from build123d import *

# Parameters (mm, degrees)
F1_DEPTH = 25.4
F3_DEPTH = 12.7
F5_DEPTH = 12.7


with BuildPart() as f1:
    # F0 (on Front) → F1 (new body)
    with BuildSketch(Plane.XZ):
        Polygon((69.85, 127), (19.05, 127), (0, 127), (0, 0), (39.624, 0), (44.45, 0), (79.248, 0), (79.248, 127), align=None)
    extrude(amount=F1_DEPTH)

    # F2 (on face) → F3 (join)
    with BuildSketch(Plane.XZ.offset(25.4)):
        with BuildLine():
            ThreePointArc((39.624, 97.79), (44.114128, 99.649872), (45.974, 104.14))
            ThreePointArc((45.974, 104.14), (35.133872, 108.630128), (39.624, 97.79))
        make_face()
    extrude(amount=F3_DEPTH)

    # F4 (on face) → F5 (cut)
    with BuildSketch(Plane(origin=(0, 0, 0), x_dir=(1, 0, 0), z_dir=(0, 0, -1))):
        with BuildLine():
            Line((16.637, 12.7), (19.812, 12.7))
            Line((19.812, 12.7), (22.987, 12.7))
            ThreePointArc((22.987, 12.7), (19.812, 15.875), (16.637, 12.7))
        make_face()
        with BuildLine():
            Line((22.987, 12.7), (19.812, 12.7))
            Line((19.812, 12.7), (16.637, 12.7))
            ThreePointArc((16.637, 12.7), (19.812, 9.525), (22.987, 12.7))
        make_face()
        with BuildLine():
            ThreePointArc((62.611, 12.7), (59.436, 15.875), (56.261, 12.7))
            Line((56.261, 12.7), (59.436, 12.7))
            Line((59.436, 12.7), (62.611, 12.7))
        make_face()
        with BuildLine():
            Line((59.436, 12.7), (56.261, 12.7))
            ThreePointArc((56.261, 12.7), (59.436, 9.525), (62.611, 12.7))
            Line((62.611, 12.7), (59.436, 12.7))
        make_face()
    extrude(amount=-F5_DEPTH, mode=Mode.SUBTRACT)


solid = f1.part
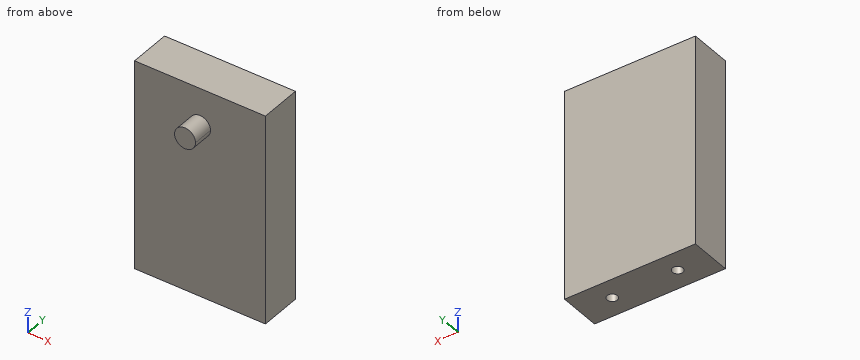
Could you check a few things on this model? Use its own coordinates, in mm. Coordinates: 2 decimals unless noted, no trailing zeros. Loops run counter-clockwise (first coordinate to the right, second up) from the corner with the lowest first, then second, coordinate; pieces in that order, holes last. Notation, with made-up numbers: (35.5, 10.25) -> (43.5, 10.25) arc R25 ccw to (43.5, 34.25) -> close; hole circle Ø6 at (72, 34). An arc over 180 degrees is marked (long way). Answer in a Markdown table with one row per item.
(1) Imagine slicing it at D-D (x = 8). List the corners of the cut face in (y, z) for me, plus the area to 3 significant figures.
Results found:
| item | result |
|---|---|
| outline | (-25.4, 0) -> (0, 0) -> (0, 127) -> (-25.4, 127) -> close |
| area | 3,230 mm^2 |
(2) Will these pins go through, and if not, where does the flat tip stop? pin 1 Ø4 at (y, z) = (-25.5, 22.5) entering from +X; pin 2 Ø1 at (x, z) = (23.5, 38) entering from -Y; pin 3 Ø1.9 at (x, y) = (20, -11.5) entering from -Z.
Results found:
| item | result |
|---|---|
| pin 1 | stops at x = 79.25 |
| pin 2 | stops at y = -25.4 |
| pin 3 | stops at z = 12.7 |
(3) Imagine slicing it at B-B (z = 63.5). List the corners of the cut face in (x, y) for me, plus the area to 3 significant figures.
Results found:
| item | result |
|---|---|
| outline | (0, -25.4) -> (79.25, -25.4) -> (79.25, 0) -> (0, 0) -> close |
| area | 2,010 mm^2 |
(4) Imagine slicing it at A-A (y = -12.7). List the corners of the cut face in (x, z) for me.
Results found:
| item | result |
|---|---|
| outline | (0, 0) -> (16.64, 0) -> (16.64, 12.7) -> (22.99, 12.7) -> (22.99, 0) -> (56.26, 0) -> (56.26, 12.7) -> (62.61, 12.7) -> (62.61, 0) -> (79.25, 0) -> (79.25, 127) -> (0, 127) -> close |
(5) If I drill on probe 1 along X at (y, z) = (-15, 7.5); probe 2 along Y at (x, z) = (18, 52.5); probe 3 along X at (y, z) = (-29.5, 106), over which ranges is the centre line in solid material (lowest first)?
Results found:
| item | result |
|---|---|
| probe 1 | x = 0 to 17.62, 22 to 57.25, 61.62 to 79.25 |
| probe 2 | y = -25.4 to 0 |
| probe 3 | x = 33.55 to 45.7 |
(6) Imagine slicing it at C-C (x = 43). List the corners of the cut face in (y, z) for me, plus the area to 3 significant figures.
Results found:
| item | result |
|---|---|
| outline | (-38.1, 98.76) -> (-25.4, 98.76) -> (-25.4, 0) -> (0, 0) -> (0, 127) -> (-25.4, 127) -> (-25.4, 109.52) -> (-38.1, 109.52) -> close |
| area | 3,360 mm^2 |
